Could you check a few things on this drawing? It's one solid part, dimensions in mm from its lowest x, y, z. Coordinates: 2 decimals unless noted, no trailing zeros. Loops run counter-clockwise (first coordinate to the right, second up) from the corner with the lowest first, then second, coordinate; pieces in that order, holes last. Notation, with made-up numbers: (9, 89.25) -> (16, 89.25) arc R35 ccw to (16, 128.25) -> close; hole circle Ø1 at (28.25, -40). An arc over 180 degrees is marked (long way). One line per question, with ' | ' between items. Start each with the question number.
(1) Suppose I cut it at D-D (y = 193). Please give me the cut outline in (x, z).
(2) Suppose I cut it at A-A (z = 76). Please give me the cut outline in (x, y), plus the area to 3 significant figures.
(3) If I drill on line 1 along Y through (x, z) = (345.5, 83.5); line 2 along Z through (x, y) = (267, 131); line 3 along X through (y, z) = (249, 41.5), over which ranges is the centre line in solid material (lowest first)?
(4) Suppose I cut it at C-C (x = 271.5). Please give me the cut outline in (y, z).
(5) I'm going to push flat-ended pins straight in: pin 1 Ø16.5 at (y, z) = (203, 114.5) entering from -X; pin 2 Ø7.5 at (y, z) = (151, 112.5) entering from -X; pin 3 Ø12.5 at (x, z) = (7, 36) entering from +Y; pin 4 Ø1.5 at (x, z) = (208, 106) entering from -Y. Where does each tip first touch, or does it pass through?
(6) Suppose I cut it at B-B (x = 89). Please give me the cut outline in (y, z).
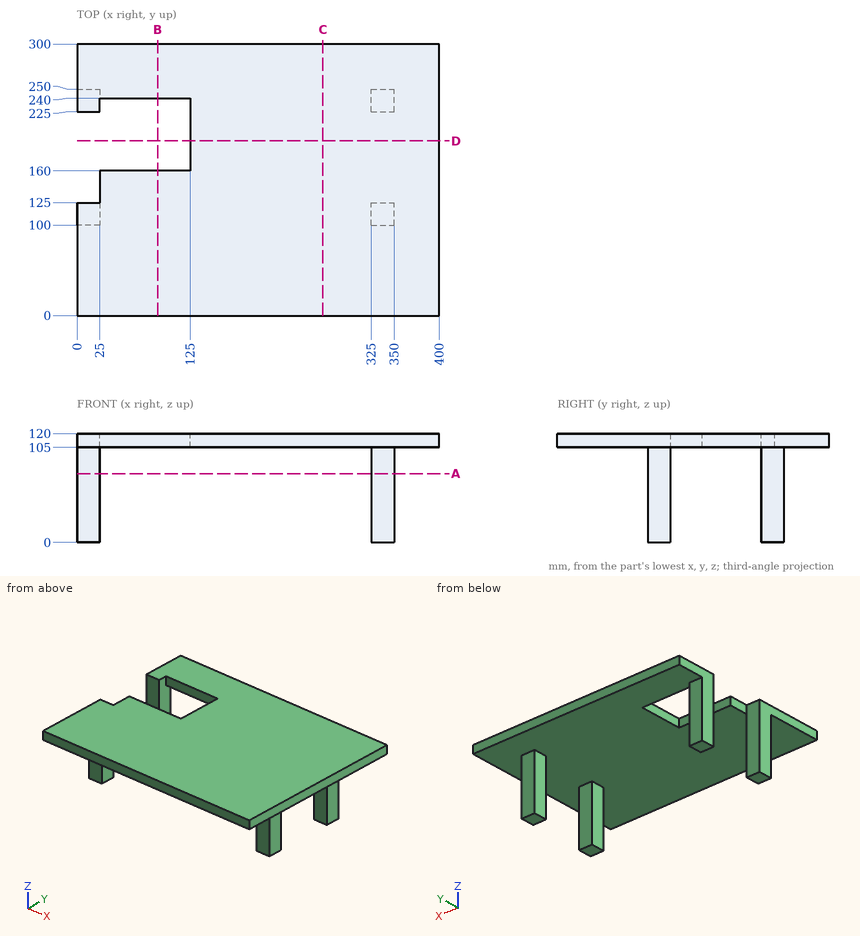
Checks:
1) outline: (125, 105) -> (400, 105) -> (400, 120) -> (125, 120) -> close
2) outline: (0, 100) -> (25, 100) -> (25, 125) -> (0, 125) -> close; (0, 225) -> (25, 225) -> (25, 250) -> (0, 250) -> close; (325, 100) -> (350, 100) -> (350, 125) -> (325, 125) -> close; (325, 225) -> (350, 225) -> (350, 250) -> (325, 250) -> close | area: 2,500 mm^2
3) line 1: y = 100 to 125, 225 to 250 | line 2: z = 105 to 120 | line 3: x = 0 to 25, 325 to 350
4) outline: (0, 105) -> (300, 105) -> (300, 120) -> (0, 120) -> close
5) pin 1: stops at x = 125 | pin 2: stops at x = 25 | pin 3: stops at y = 250 | pin 4: stops at y = 0
6) outline: (0, 105) -> (160, 105) -> (160, 120) -> (0, 120) -> close; (240, 105) -> (300, 105) -> (300, 120) -> (240, 120) -> close
